from build123d import *

# Parameters (mm, degrees)
F0_W     = 5
F0_H     = 15
F1_DEPTH = 10
F2_R     = 2.5
F3_DEPTH = 105.001
F4_R     = 4.99999
F5_W     = 95
F5_H     = 95
F6_DEPTH = 10.001


# Not quite as in the source:
# - a fillet or chamfer is up to 0.001 mm smaller than in the source, because OpenCascade refuses the exact size


with BuildPart() as f1:
    # F0 (on Top) → F1 (new body)
    with BuildSketch(Plane.XY):
        Polygon((52.5, 52.5), (-52.5, 52.5), (-52.5, -52.5), (-47.5, -52.5), (47.5, -52.5), (52.5, -52.5), align=None)
        with Locations((-50, -60)):
            Rectangle(F0_W, F0_H)
        with Locations((50, -60)):
            Rectangle(F0_W, F0_H)
    extrude(amount=F1_DEPTH)

    # F2 (on face) → F3 (cut, through all)
    with BuildSketch(Plane.YZ.offset(52.5)):
        with Locations((-62.5, 5)):
            Circle(F2_R)
    extrude(amount=-F3_DEPTH, mode=Mode.SUBTRACT)

    # F4 (radius 5 in the source; OpenCascade refuses exactly that, so slightly less here)
    f4_edges = [f1.edges().sort_by_distance(p)[0] for p in [
        (-50, -67.5, 10),
        (-50, -67.5, 0),
        (50, -67.5, 10),
        (50, -67.5, 0),
    ]]
    fillet(f4_edges, radius=F4_R)

    # F5 (on face) → F6 (cut, through all)
    with BuildSketch(Plane.XY.offset(10)):
        Rectangle(F5_W, F5_H)
    extrude(amount=-F6_DEPTH, mode=Mode.SUBTRACT)


solid = f1.part
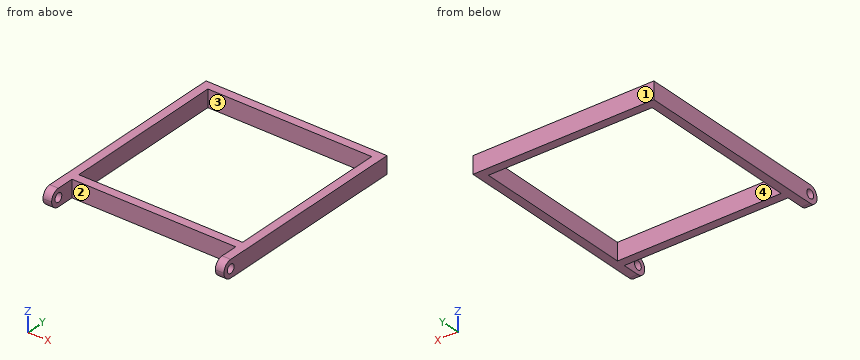
The listing builds one solid part. Answer for the finished solid, in the listing's coordinates (mm). Face numbers are marked on the shaded views. Give positions to 0.01 mm unless a question says otherwise; leave off trailing zeros. Loops run counter-clockwise (first coordinate to the right, second up) from the corner with the lowest first, then second, coordinate; pieces in that order, holes last.
Item 1: Find the intervals of material crossed by line 1 along X through (y, z) = (17.5, 6.25); line 2 along Z through (x, y) = (50.8, -62.5), in increasing order.
Derived:
line 1: x = -52.5 to -47.5, 47.5 to 52.5
line 2: z = 0 to 2.5, 7.5 to 10
Item 2: A cutting plane is placed at A-A (y = 33.5). Give the vertices of the cut face in (x, z), then the cut area to 3 significant figures.
Derived:
outline: (-52.5, 0) - (-47.5, 0) - (-47.5, 10) - (-52.5, 10) - close; (47.5, 0) - (52.5, 0) - (52.5, 10) - (47.5, 10) - close
area: 100 mm2
Item 3: This flat-tipped pin is pushed along its axis until it touches: pin 1 Ø3 at (x, z) = (-8, 4.5) entering from -Y. Where does it stop, or does it pass through?
Derived:
pin 1: stops at y = -52.5
Item 4: Determine the mould class of the marked faces 1, 2, 3 and 4 for opening direction Y: +Y half, -Y half, draft (parallel to the pull), parting line (faces both ways), or undercut.
Derived:
face 1: +Y half
face 2: -Y half
face 3: undercut
face 4: undercut
